```python
from build123d import *

# Parameters (mm, degrees)
SKETCH1_W                                = 30.83052
SKETCH1_H                                = 61.15812
BOSS_EXTRUDE1_DEPTH                      = 7.37616
SKETCH2_R                                = 9.02208
CUT_EXTRUDE1_DEPTH                       = 36.030228199
F_1_16_0_0625_DIAMETER_HOLE2_D           = 1.5875
F_1_16_0_0625_DIAMETER_HOLE2_CSINK_D     = 2.8575
F_1_16_0_0625_DIAMETER_HOLE2_CSINK_ANGLE = 90


with BuildPart() as part:
    # Sketch1 → Boss-Extrude1 (new body)
    with BuildSketch(Plane(origin=(0, 0, 0), x_dir=(1, 0, 0), z_dir=(0, 1, 0))):
        Rectangle(SKETCH1_W, SKETCH1_H)
    extrude(amount=BOSS_EXTRUDE1_DEPTH)

    # Sketch2 → Cut-Extrude1 (cut, through all)
    with BuildSketch(Plane(origin=(0, 7.37616, 0), x_dir=(1, 0, 0), z_dir=(0, 1, 0))):
        with Locations(Location((0, 0, 0), (0, 0, 270))):
            Circle(SKETCH2_R)
    extrude(amount=-CUT_EXTRUDE1_DEPTH, mode=Mode.SUBTRACT)

    # 1/16 (0.0625) Diameter Hole2 (through all)
    with Locations(Plane(origin=(0, 7.37616, 0), x_dir=(1, 0, 0), z_dir=(0, 1, 0))):
        with Locations((-11.81862, 11.684), (11.54938, 11.684), (11.81862, -11.684), (-11.81862, -11.684)):
            CounterSinkHole(F_1_16_0_0625_DIAMETER_HOLE2_D / 2, F_1_16_0_0625_DIAMETER_HOLE2_CSINK_D / 2, counter_sink_angle=F_1_16_0_0625_DIAMETER_HOLE2_CSINK_ANGLE)


solid = part.part
```
Can you work these out from the model? Positions are in its coordinate system, mm. Coordinates: 2 decimals unless noted, no trailing zeros. Loops run counter-clockwise (first coordinate to the right, second up) from the corner with the lowest first, then second, coordinate; pieces in that order, holes last. Notation, with made-up numbers: (-26.5, 26) -> (4.5, 26) arc R33 cw to (4.5, 60) -> close; hole circle Ø3 at (39.25, 83). An arc over 180 degrees is marked (long way). Answer as a JSON object with one key per item and string values.
1) Imagine slicing it at D-D (x = -12). Count the separate pieces of the cut face and the enclosed holes in it, then the cut area to 3 significant figures.
Results:
{"separate pieces": "3", "enclosed holes": "0", "area": "427 mm^2"}
2) Thinking about a two-plate mould opening in Z: for faces 1 (the face through (-7, 7.376, -7)), 2 (the face through (-8.004, 3.74, 4.163)), 3 (the face through (0, 4, 30.579)), 4 (the face through (0, 4, -30.579)), which applies, pulls with the +Z half, pulls with the -Z half, needs draft (parallel to the pull), parting line crosses it, or undercut?
Results:
{"face 1": "needs draft", "face 2": "undercut", "face 3": "pulls with the +Z half", "face 4": "pulls with the -Z half"}
3) Imagine slicing it at A-A (z = 0). Please give me the cut outline in (x, y), then the cut area to 3 significant figures.
Results:
{"outline": "(-15.42, 0) -> (-9.02, 0) -> (-9.02, 7.38) -> (-15.42, 7.38) -> close; (9.02, 0) -> (15.42, 0) -> (15.42, 7.38) -> (9.02, 7.38) -> close", "area": "94.3 mm^2"}
4) If I drill on line 1 (Z direction, x = 11.5, y = 4.25); line 2 (Z direction, x = 6.5, y = 2.25); line 3 (Z direction, x = 12, y = 1.5), over which ranges is the centre line in solid material (lowest first)?
Results:
{"line 1": "z = -30.58 to -12.48, -10.89 to 10.96, 12.41 to 30.58", "line 2": "z = -30.58 to -6.26, 6.26 to 30.58", "line 3": "z = -30.58 to -12.34, -11.03 to 10.91, 12.46 to 30.58"}
5) For P1, Ø1.4, axis at x = -11.82, z = -11.68, coming from the -Y side; P2, Ø2, axis at x = 11.82, z = 11.68, coming from the +Y side, each with a flat end and sliding along its axis, tell me the tip position at first contact or that it passes through.
Results:
{"P1": "passes through", "P2": "stops at y = 6.95"}
6) Imagine slicing it at B-B (x = 0). Please give me the cut outline in (y, z).
Results:
{"outline": "(0, -30.58) -> (7.38, -30.58) -> (7.38, -9.02) -> (0, -9.02) -> close; (0, 9.02) -> (7.38, 9.02) -> (7.38, 30.58) -> (0, 30.58) -> close"}
7) Imagine slicing it at C-C (y = 4). Please give me the cut outline in (x, z).
Results:
{"outline": "(-15.42, -30.58) -> (15.42, -30.58) -> (15.42, 30.58) -> (-15.42, 30.58) -> close; hole circle Ø1.59 at (-11.82, -11.68); hole circle Ø1.59 at (-11.82, 11.68); hole circle Ø18.04 at (0, 0); hole circle Ø1.59 at (11.55, -11.68); hole circle Ø1.59 at (11.82, 11.68)"}
